Part model, mm, in its own coordinate system. A direction names the side the tool comes from. Coordinates: 2 decimals unless noted, no trailing zeros. Order: outer loops, then holes, each group sorted by start corner. A loop starts at its lowest first (then second) coordinate and runs counter-clockwise, first axis right, second up.
from build123d import *

# Parameters (mm, degrees)
SKETCH1_R           = 7.5
SKETCH1_R_2         = 5
BOSS_EXTRUDE1_DEPTH = 4
SKETCH2_R           = 8.25
SKETCH2_R_2         = 5
BOSS_EXTRUDE2_DEPTH = 0.8
FILLET1_R           = 0.3
FILLET2_R           = 0.1


with BuildPart() as part:
    # Sketch1 → Boss-Extrude1 (new body)
    with BuildSketch(Plane(origin=(0, 0, 0), x_dir=(1, 0, 0), z_dir=(0, 1, 0))):
        with Locations(Location((0, 0, 0), (0, 0, 270))):
            Circle(SKETCH1_R)
        with Locations(Location((0, 0, 0), (0, 0, 270))):
            Circle(SKETCH1_R_2, mode=Mode.SUBTRACT)
    extrude(amount=BOSS_EXTRUDE1_DEPTH)

    # Sketch2 → Boss-Extrude2 (add)
    with BuildSketch(Plane.XZ):
        with Locations(Location((0, 0, 0), (0, 0, 270))):
            Circle(SKETCH2_R)
        with Locations(Location((0, 0, 0), (0, 0, 90))):
            Circle(SKETCH2_R_2, mode=Mode.SUBTRACT)
    extrude(amount=-BOSS_EXTRUDE2_DEPTH)

    # Fillet1
    fillet1_edges = [part.edges().sort_by_distance(p)[0] for p in [
        (0, 4, -7.5),
        (0, 0, -5),
        (0, 4, -5),
    ]]
    fillet(fillet1_edges, radius=FILLET1_R)

    # Fillet2
    fillet2_edges = [part.edges().sort_by_distance(p)[0] for p in [
        (0, 0, 8.25),
        (0, 0.8, 8.25),
    ]]
    fillet(fillet2_edges, radius=FILLET2_R)


solid = part.part
Q1. Cut at A-A on z = 0. Write the cut outline in (x, y), and give its area (3 significant figures).
Results list:
outline: (-8.25, 0.1) arc R0.1 ccw to (-8.15, 0) - (-5.3, 0) arc R0.3 ccw to (-5, 0.3) - (-5, 3.7) arc R0.3 ccw to (-5.3, 4) - (-7.2, 4) arc R0.3 ccw to (-7.5, 3.7) - (-7.5, 0.8) - (-8.15, 0.8) arc R0.1 ccw to (-8.25, 0.7) - close; (5, 0.3) arc R0.3 ccw to (5.3, 0) - (8.15, 0) arc R0.1 ccw to (8.25, 0.1) - (8.25, 0.7) arc R0.1 ccw to (8.15, 0.8) - (7.5, 0.8) - (7.5, 3.7) arc R0.3 ccw to (7.2, 4) - (5.3, 4) arc R0.3 ccw to (5, 3.7) - close
area: 21.1 mm2
Q2. Wall check: line 1 along X through (y, z) = (2.8, 0); line 2 along X through (y, z) = (2.7, -2.5); line 3 along Z through (x, y) = (2.75, 2.2). Give the ranges that are in metal, low to high.
Results list:
line 1: x = -7.5 to -5, 5 to 7.5
line 2: x = -7.07 to -4.33, 4.33 to 7.07
line 3: z = -6.98 to -4.18, 4.18 to 6.98
Q3. Cut at C-C on y = 3. Write the cut outline in (x, z).
Results list:
outline: circle Ø15 at (0, 0); hole circle Ø10 at (0, 0)
Q4. Pin check, flat tip, straight feed: pin 1 Ø2 at (y, z) = (2, 2.5) entering from -X. Stop position of the tip, or through.
Results list:
pin 1: stops at x = -7.35
Q5. Which spindle directions (+Z, -Z, +X, -X, +Y, -Y) get a long thin tool onto all of the face, cutting with end or side? Do faces 4 (the face through (0.33, 2.23, -7.493)), 5 (the face through (-5, 4, -3)). Say none if no direction does.
Results list:
face 4: +Y
face 5: +Z, -Z, +X, -X, +Y
Q6. Cut at B-B on x = 0. Write the cut outline in (y, z).
Results list:
outline: (0, -8.15) arc R0.1 ccw to (0.1, -8.25) - (0.7, -8.25) arc R0.1 ccw to (0.8, -8.15) - (0.8, -7.5) - (3.7, -7.5) arc R0.3 ccw to (4, -7.2) - (4, -5.3) arc R0.3 ccw to (3.7, -5) - (0.3, -5) arc R0.3 ccw to (0, -5.3) - close; (0, 5.3) arc R0.3 ccw to (0.3, 5) - (3.7, 5) arc R0.3 ccw to (4, 5.3) - (4, 7.2) arc R0.3 ccw to (3.7, 7.5) - (0.8, 7.5) - (0.8, 8.15) arc R0.1 ccw to (0.7, 8.25) - (0.1, 8.25) arc R0.1 ccw to (0, 8.15) - close
Q7. Mould opens along Z. For faces 1 (the face through (-4.88, 1.98, -1.08)), 2 (the face through (-5.3, 0, -1.7)), 3 (the face through (-8.054, 0.396, 1.788)) say: pulls with the +Z half, pulls with the -Z half, needs draft (parallel to the pull), parting line crosses it, or undercut.
Results list:
face 1: undercut
face 2: needs draft
face 3: parting line crosses it
